from build123d import *

# Parameters (mm, degrees)
BOSS_EXTRUDE1_DEPTH      = 2.54
BOSS_EXTRUDE1_DEPTH_BACK = 2.54
SKETCH1_R                = 2.75
BOSS_EXTRUDE2_DEPTH      = 10.16
FILLET1_R                = 2.54
SKETCH3_W                = 254
SKETCH3_H                = 12.7
BOSS_EXTRUDE3_DEPTH      = 1.27


with BuildPart() as part:
    # Sketch1 → Boss-Extrude1 (new, two sides: drawn at the far end of the back side and taken through both)
    with BuildSketch(Plane(origin=(0, 0, 0), x_dir=(1, 0, 0), z_dir=(0, 1, 0)).offset(-BOSS_EXTRUDE1_DEPTH_BACK)):
        Polygon((-146.05, -15.875), (146.05, -15.875), (146.05, 40.98799435), (127, 40.98799435), (127, 15.875), (-127, 15.875), (-127, 40.98799435), (-146.05, 40.98799435), align=None)
        with Locations(Location((-139.7, 28.252118644, 0), (0, 0, 270))):
            Circle(SKETCH1_R, mode=Mode.SUBTRACT)
        with Locations(Location((-139.7, -3.497881356, 0), (0, 0, 270))):
            Circle(SKETCH1_R, mode=Mode.SUBTRACT)
        with Locations(Location((139.7, -3.497881356, 0), (0, 0, 270))):
            Circle(SKETCH1_R, mode=Mode.SUBTRACT)
        with Locations(Location((139.7, 28.252118644, 0), (0, 0, 270))):
            Circle(SKETCH1_R, mode=Mode.SUBTRACT)
        with Locations(Location((5.588, 9.525, 0), (0, 0, 270))):
            Circle(SKETCH1_R, mode=Mode.SUBTRACT)
        with Locations(Location((-121.412, 9.525, 0), (0, 0, 270))):
            Circle(SKETCH1_R, mode=Mode.SUBTRACT)
    extrude(amount=BOSS_EXTRUDE1_DEPTH + BOSS_EXTRUDE1_DEPTH_BACK)

    # Sketch2 → Boss-Extrude2 (add)
    with BuildSketch(Plane(origin=(0, 2.54, 0), x_dir=(1, 0, 0), z_dir=(0, 1, 0))):
        with BuildLine():
            Line((-139.7, 33.332118644), (-139.7, 40.98799435))
            Line((-139.7, 40.98799435), (-146.05, 40.98799435))
            Line((-146.05, 40.98799435), (-146.05, 12.556497175))
            Line((-146.05, 12.556497175), (-139.7, 12.556497175))
            Line((-139.7, 12.556497175), (-139.7, 23.172118644))
            ThreePointArc((-139.7, 23.172118644), (-144.78, 28.252118644), (-139.7, 33.332118644))
        make_face()
        with BuildLine():
            Line((146.05, 40.98799435), (146.05, 12.556497175))
            Line((146.05, 12.556497175), (139.7, 12.556497175))
            Line((139.7, 12.556497175), (139.7, 23.172118644))
            ThreePointArc((139.7, 23.172118644), (144.78, 28.252118644), (139.7, 33.332118644))
            Line((139.7, 33.332118644), (139.7, 40.98799435))
            Line((139.7, 40.98799435), (146.05, 40.98799435))
        make_face()
    extrude(amount=BOSS_EXTRUDE2_DEPTH)

    # Fillet1
    fillet1_edges = [part.edges().sort_by_distance(p)[0] for p in [
        (142.875, 2.54, -12.556497175),
        (146.05, 7.62, -12.556497175),
        (-146.05, 2.54, 1.659251412),
        (-146.05, 5.08, -40.98799435),
        (146.05, 5.08, -40.98799435),
        (146.05, 2.54, 1.659251412),
        (-142.875, 2.54, -12.556497175),
        (-146.05, 7.62, -12.556497175),
    ]]
    fillet(fillet1_edges, radius=FILLET1_R)

    # Sketch3 → Boss-Extrude3 (add)
    with BuildSketch(Plane(origin=(0, 2.54, 0), x_dir=(1, 0, 0), z_dir=(0, 1, 0))):
        with Locations((0, -9.525)):
            Rectangle(SKETCH3_W, SKETCH3_H)
    extrude(amount=BOSS_EXTRUDE3_DEPTH)


solid = part.part
Check sheet for the modelled part. Datum: model origin and axes. Units: mm. A direction names the side the tool comes from. Round coordinates to 2 decimals unless told otherwise and drop trailing zeros. Order: outer loops, then holes, each group sorted by start corner. A loop starts at its lowest first (then second) coordinate and runs counter-clockwise, first axis right, second up. Notation, with made-up numbers: M 1,39 L 25,39 A22 ccw 25,64 Z; hole C 28.25,76.25 d9. An arc over 180 degrees is marked long. One line per item, written item: value. Start each with the question number.
1. Section check A-A on y = 10. Enter the section's corners in (x, z), and give its area (3 significant figures).
2. Access from +Z, -Z, +X, -X, +Y, -Y to the whole of each face (thin tool, end or side, straight path). Record for faces 1 (the flat face through (127, 0, -29)), 2 (the cylindrical face through (-142.385, -0.036, -28.848)), 3 (the flat face through (-139.7, 8, -18)), 4 (the cylindrical face through (-144.78, 7.55, -28.14)).
3. Gauge pin test, flat ends, axial feed: P1, Ø1.1, axis at x = 142, y = 8, coming from the +Z side; P2, Ø3.5, axis at x = -121.412, z = -9.525, coming from the +Y side; P3, Ø1.4, axis at y = 3.5, z = 11, coming from the -X side; P4, Ø3, axis at x = 75.5, z = -16.5, coming from the +Y side. Record the tip position at first contact, or that the pin passes through.
4. Section check C-C on x = 48. Enter the section's corners in (y, z) (3 decimals).
5. Section check B-B on z = -28.5. Enter the section's corners in (x, y), and give its area (3 significant figures).
6. Release check for a two-part mould opening along X. For faces 5 (the flat face through (-145, 12.7, -27)), 6 (the flat face through (146.05, 3, -23)), 7 (the cylindrical face through (-142.385, -0.036, 2.902)) record: released by +X, released by -X, zero draft, split by the parting line, or undercut.
7. Scan lines: line 1 along Z through (x, y) = (-139.7, 0.1) (3 decimals); line 2 along X through (y, z) = (-1.25, 3.5); line 3 along X through (y, z) = (10.75, -20). Record each from-to range of solid material in increasing order.
Results found:
1. outline: M -146.05,-38.45 A2.54 ccw -143.51,-40.99 L -139.7,-40.99 L -139.7,-33.33 A5.08 cw -139.7,-23.17 L -139.7,-12.56 L -143.51,-12.56 A2.54 ccw -146.05,-15.1 Z; M 139.7,-40.99 L 143.51,-40.99 A2.54 ccw 146.05,-38.45 L 146.05,-15.1 A2.54 ccw 143.51,-12.56 L 139.7,-12.56 L 139.7,-23.17 A5.08 cw 139.7,-33.33 Z
1. area: 274 mm^2
2. face 1: -Z, +Y, -Y
2. face 2: +Y, -Y
2. face 3: +Z, -Z, +Y
2. face 4: +Y
3. P1: z = -12.56
3. P2: through
3. P3: x = -127
3. P4: y = 2.54
4. outline: M -2.54,-15.875 L 2.54,-15.875 L 2.54,3.175 L 3.81,3.175 L 3.81,15.875 L -2.54,15.875 Z
5. outline: M -146.05,-2.54 L -142.44,-2.54 L -142.44,2.54 L -144.77,2.54 L -144.77,12.7 L -146.05,12.7 Z; M -136.96,-2.54 L -127,-2.54 L -127,2.54 L -136.96,2.54 Z; M 127,-2.54 L 136.96,-2.54 L 136.96,2.54 L 127,2.54 Z; M 142.44,-2.54 L 146.05,-2.54 L 146.05,12.7 L 144.77,12.7 L 144.77,2.54 L 142.44,2.54 Z
5. area: 164 mm^2
6. face 5: zero draft
6. face 6: released by +X
6. face 7: undercut
7. line 1: -40.988 to -31.002, -25.502 to 0.748, 6.248 to 15.875
7. line 2: -146.05 to -142.45, -136.95 to 136.95, 142.45 to 146.05
7. line 3: -146.05 to -139.7, 139.7 to 146.05
